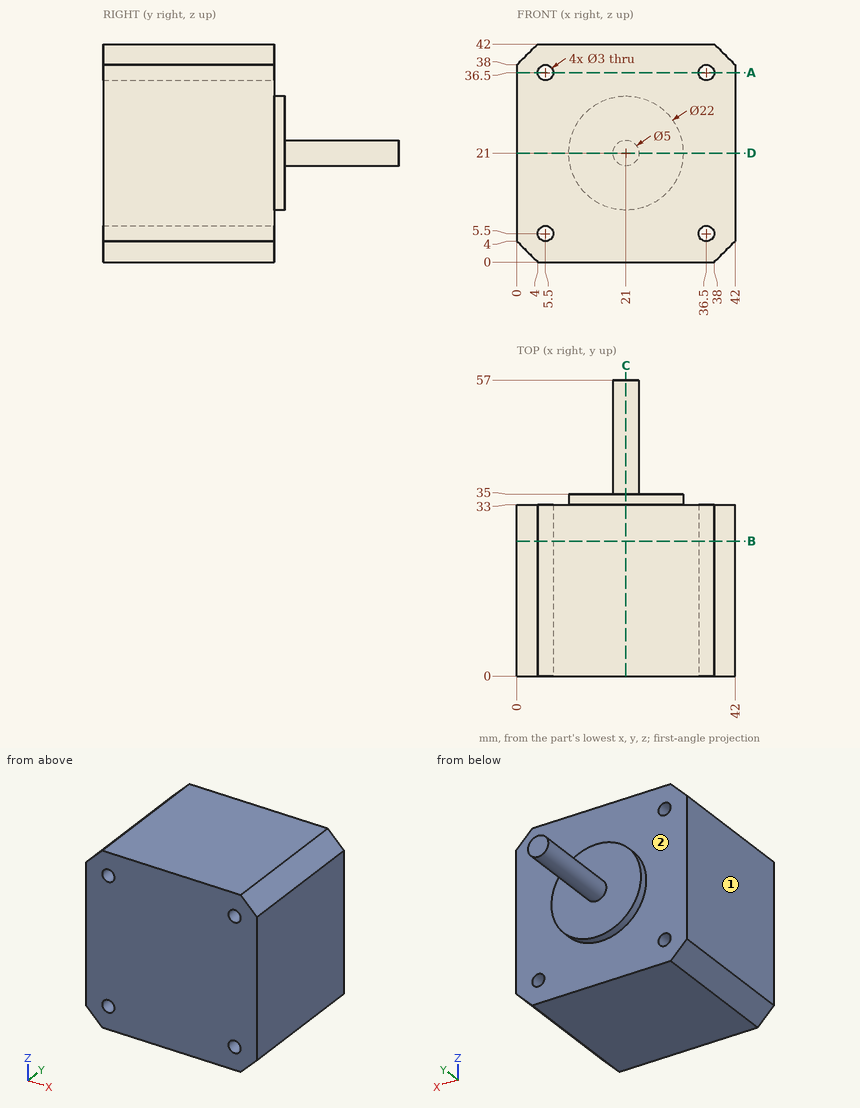
Answer from the drawing. Dimensions are ordinates in mm from the lowest x, y and z of the part. A direction names the side the tool comes from. Give positions to 0.01 mm unless a question says otherwise; leave off trailing zeros. Write each loop counter-clockwise with the first axis right and the second up, starting at its lowest first coordinate (ties: lowest second). Pieces come first, ordered by that corner, then holes. Notation, with made-up numbers: (40, 61.5) -> (83, 61.5) arc R25 cw to (83, 91.5) -> close; hole circle Ø8 at (-30.5, 64). An arc over 180 degrees is marked (long way). One line per question, with ' | ' between items. Start each with the question number.
1. Section C-C (x = 21) is taken. Determine the outline of the cut face in (y, z), plus the area to 3 significant figures.
2. Section B-B (y = 26) is taken. Determine the outline of the cut face in (x, z).
3. Section A-A (z = 36.5) is taken. Determine the outline of the cut face in (x, y).
4. Find the intervals of material crossed by probe 1 along X at (y, z) = (8, 5.5); probe 2 along X at (y, z) = (32, 6), in increasing order.
5. Given pin 1 Ø21 at (x, z) = (11, 30.5) entering from +Y; pin 2 Ø8 at (y, z) = (47.5, 15.5) entering from -X; pin 3 Ø3 at (x, z) = (14.5, 6) entering from +Y, each flat-ended and moving along its own axis, determine where each tip first touches the part or whether it passes through.
6. Section D-D (z = 21) is taken. Determine the outline of the cut face in (x, y).
7. For the marked faces 1 and 2, determine the directions among +Z, -Z, +X, -X, +Y, -Y from which every point of the face is accessible in a straight line to the end or side of a thin tool.
Response values:
1) outline: (0, 0) -> (33, 0) -> (33, 10) -> (35, 10) -> (35, 18.5) -> (57, 18.5) -> (57, 23.5) -> (35, 23.5) -> (35, 32) -> (33, 32) -> (33, 42) -> (0, 42) -> close | area: 1,540 mm2
2) outline: (0, 4) -> (4, 0) -> (38, 0) -> (42, 4) -> (42, 38) -> (38, 42) -> (4, 42) -> (0, 38) -> close; hole circle Ø3 at (5.5, 5.5); hole circle Ø3 at (5.5, 36.5); hole circle Ø3 at (36.5, 5.5); hole circle Ø3 at (36.5, 36.5)
3) outline: (0, 0) -> (4, 0) -> (4, 33) -> (0, 33) -> close; (7, 0) -> (35, 0) -> (35, 33) -> (7, 33) -> close; (38, 0) -> (42, 0) -> (42, 33) -> (38, 33) -> close
4) probe 1: 0 to 4, 7 to 35, 38 to 42 | probe 2: 0 to 4.09, 6.91 to 35.09, 37.91 to 42
5) pin 1: y = 35 | pin 2: x = 19 | pin 3: y = 33
6) outline: (0, 0) -> (42, 0) -> (42, 33) -> (32, 33) -> (32, 35) -> (23.5, 35) -> (23.5, 57) -> (18.5, 57) -> (18.5, 35) -> (10, 35) -> (10, 33) -> (0, 33) -> close
7) face 1: +Z, -Z, -X, +Y, -Y | face 2: +Y
